```python
from build123d import *

# Parameters (mm, degrees)
SKETCH1_R           = 4
BOSS_EXTRUDE1_DEPTH = 6.5
CHAMFER1_SIZE       = 0.25


with BuildPart() as part:
    # Sketch1 → Boss-Extrude1 (new body)
    with BuildSketch(Plane.XY):
        Polygon((7.1, 0), (3.55, 6.148780367), (-3.55, 6.148780367), (-7.1, 0), (-3.55, -6.148780367), (3.55, -6.148780367), align=None)
        with Locations(Location((0, 0, 0), (0, 0, 180))):
            Circle(SKETCH1_R, mode=Mode.SUBTRACT)
    extrude(amount=BOSS_EXTRUDE1_DEPTH)

    # Chamfer1
    chamfer1_edges = [part.edges().sort_by_distance(p)[0] for p in [
        (4, 0, 0),
        (4, 0, 6.5),
    ]]
    chamfer(chamfer1_edges, length=CHAMFER1_SIZE)

    # Sketch3 → Cut-Revolve1 (revolve, cut)
    with BuildSketch(Plane(origin=(0, 0, 0), x_dir=(1, 0, 0), z_dir=(0, 1, 0)), mode=Mode.PRIVATE) as cut_revolve1_sk:
        Polygon((-1, -7.5), (-4.429629983, -7.5), (-8, -5), (-8, -1.5), (-4.429629983, 1), (-1, 1), (-1, 1.925478013), (-9.540810572, 1.925478013), (-9.540810572, -8.900626742), (-1, -8.900626742), align=None)
    revolve(cut_revolve1_sk.sketch.rotate(Axis((0, 0, 7.5), (0, 0, -1)), 180), axis=Axis((0, 0, 7.5), (0, 0, -1)), mode=Mode.SUBTRACT)


solid = part.part
```
Here's how the part is built. I have some questions about the finished solid (model axes, mm). Give positions to 0.01 mm unless a question says otherwise; leave off trailing zeros. Write each loop counter-clockwise with the first axis right and the second up, starting at its lowest first coordinate (ties: lowest second). Pieces come first, ordered by that corner, then holes. Notation, with made-up numbers: M 30.25,29 L 44.25,29 A17 ccw 44.25,46 Z; hole C -40,-23.75 d9. An arc over 180 degrees is marked long. Put each result on its own line as item: value. Start each with the question number.
Item 1: I need wall thicknesses on L1, parallel to Y at x = 0, z = 2.1; L2, parallel to X at y = 2, z = 1; L3, parallel to X at y = 3.5, z = 1.25. Which ranges of each line are inside material? Lowest first, please. Write a range as from..to.
Item 2: Will this pin go through, and if not, where does the flat tip stop? pin 1 (1.5 mm diameter, centred on y = 3, z = 3.5, fed in from +X).
Item 3: If we section it at B-B, the plane x = 0: Write out the boundary of the cut face in (y, z).
Item 4: Thinking about a two-plate mould opening in X: for faces 1 (the cylindrical face through (0.867, 3.905, 3.208)), 2 (the flat face through (5.35, 3.03, 3.21)), 3 (the flat face through (0, 6.149, 3)), 4 (the flat face through (-5.3, 3.12, 3.21)), which applies, +X half, -X half, draft (parallel to the pull), parting line (faces both ways), or undercut?
Item 5: If we section it at A-A, the plane z = 3: Write out the boundary of the cut face in (x, y).
Values:
1. L1: -6.15..-4, 4..6.15
1. L2: -5.95..-3.46, 3.46..5.95
1. L3: -5.08..-1.94, 1.94..5.08
2. pin 1: x = 5.8
3. outline: M -6.15,0.2 L -5.86,0 L -4.25,0 L -4,0.25 L -4,6.25 L -4.25,6.5 L -5.86,6.5 L -6.15,6.3 Z; M 4,0.25 L 4.25,0 L 5.86,0 L 6.15,0.2 L 6.15,6.3 L 5.86,6.5 L 4.25,6.5 L 4,6.25 Z
4. face 1: undercut
4. face 2: +X half
4. face 3: draft
4. face 4: -X half
5. outline: M -7.1,0 L -3.55,-6.15 L 3.55,-6.15 L 7.1,0 L 3.55,6.15 L -3.55,6.15 Z; hole C 0,0 d8
